Verification items for this drawing (mm, ordinates from the low corner). Give positions to 0.01 mm unless a question says otherwise; leave off trailing zeros. Loops run counter-clockwise (first coordinate to the right, second up) from the corner with the lowest first, then second, coordinate; pieces in that order, holes last. Notation, with made-up numbers: (66.5, -19) -> (101.5, -19) arc R16 ccw to (101.5, -8) -> close; hole circle Ø6 at (11, 74.5). An arc over 180 degrees is marked (long way). Answer as a JSON object with one key per item and string values.
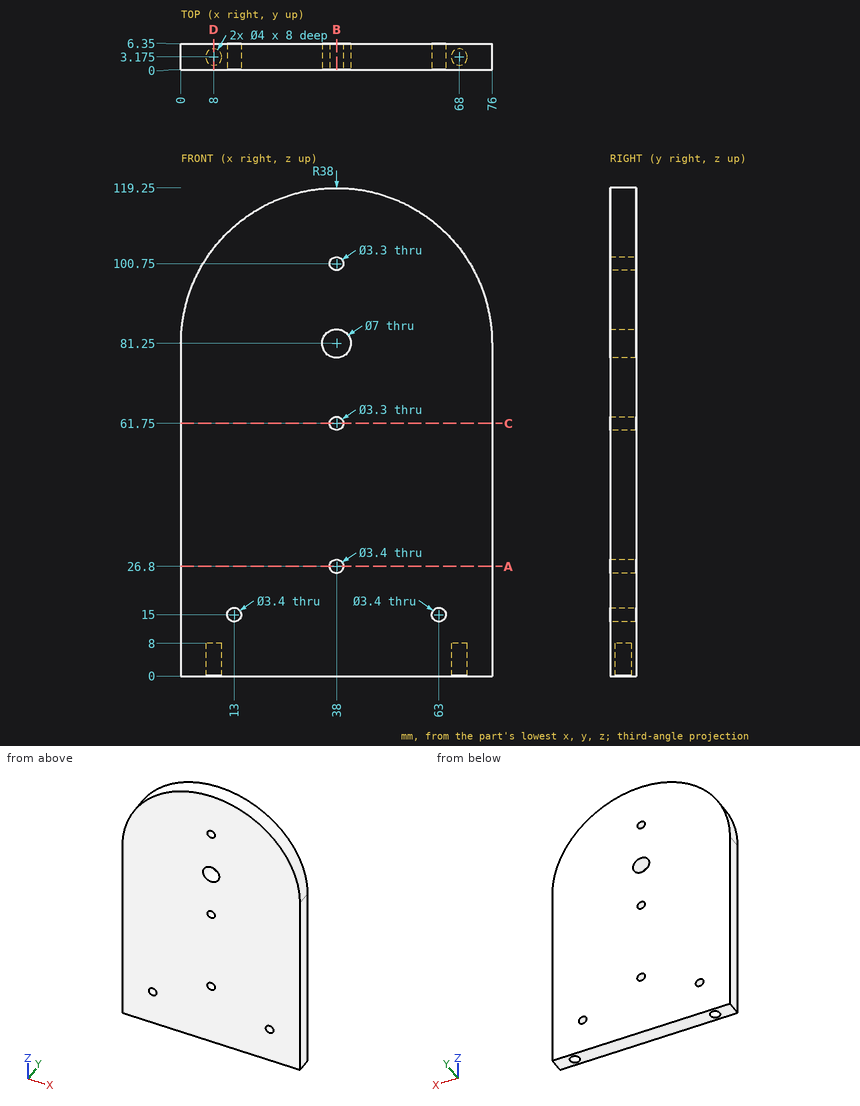
1) Section check A-A on z = 26.8. Record the cut outline in (x, y), plus the area to 3 significant figures.
Geometry check:
{"outline": "(0, 0) -> (36.3, 0) -> (36.3, 6.35) -> (0, 6.35) -> close; (39.7, 0) -> (76, 0) -> (76, 6.35) -> (39.7, 6.35) -> close", "area": "461 mm2"}
2) Section check C-C on z = 61.75. Record the cut outline in (x, y).
Geometry check:
{"outline": "(0, 0) -> (36.35, 0) -> (36.35, 6.35) -> (0, 6.35) -> close; (39.65, 0) -> (76, 0) -> (76, 6.35) -> (39.65, 6.35) -> close"}
3) Section check B-B on x = 38. Record the cut outline in (y, z).
Geometry check:
{"outline": "(0, 0) -> (6.35, 0) -> (6.35, 25.1) -> (0, 25.1) -> close; (0, 28.5) -> (6.35, 28.5) -> (6.35, 60.1) -> (0, 60.1) -> close; (0, 63.4) -> (6.35, 63.4) -> (6.35, 77.75) -> (0, 77.75) -> close; (0, 84.75) -> (6.35, 84.75) -> (6.35, 99.1) -> (0, 99.1) -> close; (0, 102.4) -> (6.35, 102.4) -> (6.35, 119.25) -> (0, 119.25) -> close"}
4) Material ranges on line 1 along X through (y, z) = (2.75, 15); line 2 along Y through (x, z) = (68, 4.5) (3 decimals); line 3 along X through (y, z) = (3.25, 81), recorded low to high. Write a range as from..to.
Geometry check:
{"line 1": "x = 0..11.3, 14.7..61.3, 64.7..76", "line 2": "y = 0..1.175, 5.175..6.35", "line 3": "x = 0..34.51, 41.49..76"}
5) Depth check by flat-ended pin: P1, Ø3, axis at x = 16.5, y = 4.5, coming from the +Z side; P2, Ø3.5, axis at x = 68, y = 3.175, coming from the +Z side; P3, Ø3, axis at x = 68, y = 3, coming from the -Z side; P4, Ø2, axis at x = 63, z = 15, coming from the -Y side. Enter the tip coordinate at first touch or a pass-through.
Geometry check:
{"P1": "stops at z = 113.56", "P2": "stops at z = 106.67", "P3": "stops at z = 8", "P4": "passes through"}
6) Section check D-D on x = 8. Record the cut outline in (y, z) (3 decimals).
Geometry check:
{"outline": "(0, 0) -> (1.175, 0) -> (1.175, 8) -> (5.175, 8) -> (5.175, 0) -> (6.35, 0) -> (6.35, 104.574) -> (0, 104.574) -> close"}
